```python
from build123d import *

# Parameters (mm, degrees)
EXTRUDE_3_DEPTH     = 15
EXTRUDE_4_DEPTH     = 4
SKETCH_8_R          = 1.6
CUT_EXTRUDE_1_DEPTH = 27.665153141


with BuildPart() as part:
    # Sketch 3 → Extrude 3 (new body)
    with BuildSketch(Plane(origin=(0, 0, 0), x_dir=(1, 0, 0), z_dir=(0, 1, 0))):
        with BuildLine():
            Line((1.616451797, 11.860683611), (-6.383548203, 11.860683611))
            Line((-6.383548203, 11.860683611), (-6.383548203, 9.575683611))
            Line((-6.383548203, 9.575683611), (1.331451797, 9.575683611))
            Line((1.331451797, 9.575683611), (1.331451797, -0.924316389))
            Line((1.331451797, -0.924316389), (-6.383548203, -0.924316389))
            Line((-6.383548203, -0.924316389), (-6.383548203, -3.209316389))
            Line((-6.383548203, -3.209316389), (1.616451797, -3.209316389))
            ThreePointArc((1.616451797, -3.209316389), (3.030665359, -2.623529952), (3.616451797, -1.209316389))
            Line((3.616451797, -1.209316389), (3.616451797, 9.860683611))
            ThreePointArc((3.616451797, 9.860683611), (3.030665359, 11.274897173), (1.616451797, 11.860683611))
        make_face()
    extrude(amount=EXTRUDE_3_DEPTH)

    # Sketch 3_4 → Extrude 4 (add)
    with BuildSketch(Plane(origin=(0, 0, 0), x_dir=(1, 0, 0), z_dir=(0, 1, 0))):
        Polygon((3.616451797, 14.325683611), (3.616451797, 9.860683611), (3.616451797, -1.209316389), (3.616451797, -5.674316389), (19.616451797, -5.674316389), (19.616451797, 14.325683611), align=None)
    extrude(amount=EXTRUDE_4_DEPTH)

    # Sketch 8 → Cut-Extrude 1 (cut, through all)
    with BuildSketch(Plane(origin=(0, 4, 0), x_dir=(1, 0, 0), z_dir=(0, 1, 0))):
        with Locations(Location((7.316451797, 7.325683611, 0), (0, 0, 270))):
            Circle(SKETCH_8_R)
        with Locations(Location((15.916451797, 7.325683611, 0), (0, 0, 270))):
            Circle(SKETCH_8_R)
    extrude(amount=-CUT_EXTRUDE_1_DEPTH, mode=Mode.SUBTRACT)


solid = part.part
```
Can you work these out from the model? Positions are in its coordinate system, mm. A direction names the side the tool comes from. Coordinates: 2 decimals unless noted, no trailing zeros. Loops run counter-clockwise (first coordinate to the right, second up) from the corner with the lowest first, then second, coordinate; pieces in that order, holes last. Notation, with made-up numbers: (-12, 2.5) - (41, 2.5) arc R20 ccw to (41, 34.5) - close; hole circle Ø9 at (86, 56.5). An arc over 180 degrees is marked (long way). Answer as CSV lines item,"result". Start each with the question number.
1) Suppose I cut it at B-B (z = 2.25). Please give me the cut outline in (x, y), plus the area to 3 significant figures.
2) For pin 1 (4 mm diameter, centred on x = -0.5, y = 5, fed in from -Z); pin 2 (5 mm diameter, centred on y = 8.5, z = -2, fed in from -X); pin 3 (2.5 mm diameter, centred on x = -3, y = 4.5, fed in from +Z), each with a flat end and sliding along its axis, tell me the tip position at first contact or that it passes through.
3) Suppose I cut it at A-A (x = -0.75). Please give me the cut outline in (y, z).
4) Which directions (+Z, -Z, +X, -X, +Y, -Y) give clear straight access to the entire face, cutting with the end or side of a thin tool? Please do faces 1 (the flat face through (12, 4, -4)), 2 (the flat face through (2, 15, -4)), 3 (the flat face through (-2, 7, -11.861)), 4 (the flat face through (-3, 7, -9.576)).
5) Suppose I cut it at D-D (z = -7). Please give me the cut outline in (x, y), plus the area to 3 significant figures.
6) I need wall thicknesses on line 1 (Z direction, x = -1.75, y = 4); line 2 (Y direction, x = 18.25, z = 2.5); line 3 (X direction, y = 8.25, z = -0.5). Which ranges of each line are inside material? Lowest first, please. Write a range as from..to.
7) Thinking about a two-plate mould opening in Z: for faces 5 (the flat face through (-2, 7, 3.209)), 6 (the flat face through (-6.384, 7, 2)), 7 (the flat face through (-2, 7, 0.924)), which applies, pulls with the +Z half, pulls with the -Z half, needs draft (parallel to the pull), parting line crosses it, or undercut?
8) Suppose I cut it at C-C (y = 11.75). Please give me the cut outline in (x, z), plus the area to 3 significant figures.
Check result:
1,outline,"(-6.38, 0) - (3.32, 0) - (3.32, 15) - (-6.38, 15) - close; (3.62, 0) - (19.62, 0) - (19.62, 4) - (3.62, 4) - close"
1,area,"210 mm²"
2,pin 1,"stops at z = -11.86"
2,pin 2,"stops at x = 1.33"
2,pin 3,"stops at z = 3.21"
3,outline,"(0, -11.86) - (15, -11.86) - (15, -9.58) - (0, -9.58) - close; (0, 0.92) - (15, 0.92) - (15, 3.21) - (0, 3.21) - close"
4,face 1,"+Z, -Z, +X, +Y"
4,face 2,"+Z, -Z, +X, -X, +Y"
4,face 3,"-Z, -X, +Y, -Y"
4,face 4,"-X, +Y, -Y"
5,outline,"(1.33, 0) - (5.75, 0) - (5.75, 4) - (3.62, 4) - (3.62, 15) - (1.33, 15) - close; (8.88, 0) - (14.35, 0) - (14.35, 4) - (8.88, 4) - close; (17.48, 0) - (19.62, 0) - (19.62, 4) - (17.48, 4) - close"
5,area,"73.2 mm²"
6,line 1,"z = -11.86..-9.58, 0.92..3.21"
6,line 2,"y = 0..4"
6,line 3,"x = 1.33..3.62"
7,face 5,"pulls with the +Z half"
7,face 6,"needs draft"
7,face 7,"undercut"
8,outline,"(-6.38, -11.86) - (1.62, -11.86) arc R2 ccw to (3.62, -9.86) - (3.62, 1.21) arc R2 ccw to (1.62, 3.21) - (-6.38, 3.21) - (-6.38, 0.92) - (1.33, 0.92) - (1.33, -9.58) - (-6.38, -9.58) - close"
8,area,"68.0 mm²"
